```python
from build123d import *

# Parameters (mm, degrees)
BOSS_EXTRUDE1_DEPTH = 5
HOLES_R             = 1.650876527
HOLES_R_2           = 1.650891558
CUT_EXTRUDE1_DEPTH  = 36.37184843


with BuildPart() as part:
    # outline → Boss-Extrude1 (new body)
    with BuildSketch(Plane.XY):
        Polygon((0.012852413, 8.079831137), (12.627409632, 8.079831137), (12.627409632, 5.682741476), (25.630939629, 5.682741476), (25.630939629, 8.079831137), (28.565803795, 8.079831137), (34.071747683, 6.239460073), (34.071747683, -0.017512268), (0, 0), align=None)
    extrude(amount=-BOSS_EXTRUDE1_DEPTH)

    # holes → Cut-Extrude1 (cut, through all)
    with BuildSketch(Plane.XY):
        with Locations((4.673381995, 4.809052053)):
            Circle(HOLES_R)
        with Locations((29.983123795, 4.809407398)):
            Circle(HOLES_R_2)
    extrude(amount=-CUT_EXTRUDE1_DEPTH, mode=Mode.SUBTRACT)


solid = part.part
```
The model under review builds one solid part; all positions refer to its coordinate system, in mm. A direction names the side the tool comes from. Round coordinates to 2 decimals unless told otherwise and drop trailing zeros. Write each loop counter-clockwise with the first axis right and the second up, starting at its lowest first coordinate (ties: lowest second). Pieces come first, ordered by that corner, then holes. Notation, with made-up numbers: M -39,76 L -28,76 A34 ccw -28,106 Z; hole C 35,38.5 d6. An arc over 180 degrees is marked long. Use CSV: the item, a comma, the result in double quotes. Start each with the question number.
(1) We need section A-A, the plane y = 4. State the section outline as (x, z) points, then the cut area to 3 significant figures.
(2) Tool access review of faces 1 (the face through (12.627, 7, -2)), 2 (the face through (31.28, 7.173, -2.465)): name each direction out of +Z, -Z, +X, -X, +Y, -Y from which nothing blocks a thin tool from reaching the whole face with its end or side.
(3) The part is to be moulded in two halves that separate along Y. For faces 3 (the face through (17, 3, 0)), 4 (the face through (31.558, 5.305, -2.465)), 5 (the face through (6, 8.08, -2)), say which applies: +Y half, -Y half, draft (parallel to the pull), parting line (faces both ways), or undercut.
(4) We need section B-B, the plane z = -4.1. State the section outline as (x, y) points, then the cut area to 3 significant figures.
(5) We need section D-D, the plane x = 20.5. State the section outline as (y, z) points, then the cut area to 3 significant figures.
(6) For line 1 along X through (y, z) = (4.5, -4.25); line 2 along X through (y, z) = (5, -1.8); line 3 along X through (y, z) = (1.5, -1.3), list the stretches that pass through material, from the lowest coordinate up.
(7) Clearance check with flat-ended pins moving along their axes: P1, Ø2.5, axis at x = 22, z = -1.5, coming from the +Y side; P2, Ø1.2, axis at y = 7, z = -3.5, coming from the -X side. State where each tip first meets the part, or that it passes through.
(8) We need section C-C, the plane x = 6. State the section outline as (y, z) points, then the cut area to 3 significant figures.
Findings:
1,outline,"M 0.01,-5 L 3.23,-5 L 3.23,0 L 0.01,0 Z; M 6.11,-5 L 28.54,-5 L 28.54,0 L 6.11,0 Z; M 31.42,-5 L 34.07,-5 L 34.07,0 L 31.42,0 Z"
1,area,"142 mm^2"
2,face 1,"+Z, -Z, +Y"
2,face 2,"+Z, -Z, +X, +Y"
3,face 3,"draft"
3,face 4,"undercut"
3,face 5,"+Y half"
4,outline,"M 0,0 L 34.07,-0.02 L 34.07,6.24 L 28.57,8.08 L 25.63,8.08 L 25.63,5.68 L 12.63,5.68 L 12.63,8.08 L 0.01,8.08 Z; hole C 4.67,4.81 d3.3; hole C 29.98,4.81 d3.3"
4,area,"222 mm^2"
5,outline,"M -0.01,-5 L 5.68,-5 L 5.68,0 L -0.01,0 Z"
5,area,"28.5 mm^2"
6,line 1,"0.01 to 3.05, 6.3 to 28.36, 31.6 to 34.07"
6,line 2,"0.01 to 3.03, 6.31 to 28.34, 31.62 to 34.07"
6,line 3,"0 to 34.07"
7,P1,"y = 5.68"
7,P2,"x = 0.01"
8,outline,"M 0,-5 L 3.83,-5 L 3.83,0 L 0,0 Z; M 5.79,-5 L 8.08,-5 L 8.08,0 L 5.79,0 Z"
8,area,"30.6 mm^2"
